Geometry: final body of the model. Coordinates: model frame, mm. A direction names the side the tool comes from. Give positions to 0.01 mm unless a question says otherwise; leave off trailing zeros. Write each loop counter-clockwise with the first axis right and the second up, starting at its lowest first coordinate (ties: lowest second). Pieces come first, ordered by that corner, then holes. Notation, with made-up numbers: M 15.5,80.5 L 65.5,80.5 A18 ccw 65.5,114.5 Z; hole C 26.25,48 d11. An arc over 180 degrees is marked long. Use one line per item in the form item = value. Start each with the question number.
Item 1: Contact query for flat-ended pins moving along their axis: P1, Ø1.5, axis at x = -25.5, y = -13.5, coming from the +Z side; P2, Ø8, axis at x = -6.5, y = -26.5, coming from the -Z side; P3, Ø3, axis at x = -5, y = -24, coming from the -Z side; P4, Ø1, axis at y = -25.5, z = -6.5, coming from the +X side. Output: stop coordinate, or through.
Item 2: Access query for faces 1 (the flat face through (-27, -12, 15)), 2 (the flat face through (-11, -20, -10)), 3 (the flat face through (-11, -20, -15)). Directions: +Z, -Z, +X, -X, +Y, -Y. A direction counts if a zero-diameter tool reaches every point of the face in a straight line with its end or side. Return the directions, or none.
Item 3: Section query D-D on y = -16. Return loops of the section in (x, z).
Item 4: Section query C-C on x = -25.5. Return loops of the section in (y, z).
Item 5: Section query A-A on y = -23. Return loops of the section in (x, z).
Item 6: Section query B-B on z = -12. Return loops of the section in (x, y).
Item 7: Material intervals for line 1 along Y through (x, z) = (16, 1); line 2 along X through (y, z) = (-17.5, -0.5); line 3 along Z through (x, y) = (-16.5, -13), sorted ascending. Write a range as from..to.
from build123d import *

# Parameters (mm, degrees)
F1_DEPTH = 10
F0_W     = 30
F0_H     = 5
F2_DEPTH = 35
F4_DEPTH = 10.001
F6_DEPTH = 10.001


with BuildPart() as f1:
    # F0 (on Front) → F1 (new body)
    with BuildSketch(Plane.XZ):
        Polygon((32.5, 0), (-7.5, 20), (-22.5, 20), (-32.5, 20), (-32.5, 15), (-22.5, 15), (-22.5, -10), (7.5, -10), (7.5, -15), (-22.5, -15), (-22.5, -20), (32.5, -20), align=None)
    extrude(amount=F1_DEPTH)

    # F0 (on Front) → F2 (join)
    with BuildSketch(Plane.XZ):
        Polygon((-22.5, 15), (-32.5, 15), (-32.5, 10), (-32.5, -20), (-22.5, -20), (-22.5, -15), (-22.5, -10), align=None)
        with Locations((-7.5, -12.5)):
            Rectangle(F0_W, F0_H)
    extrude(amount=F2_DEPTH)

    # F3 (on face) → F4 (cut, through all)
    with BuildSketch(Plane.XY.offset(-10)):
        Polygon((7.5, -10), (-22.5, -35), (7.5, -35), align=None)
    extrude(amount=-F4_DEPTH, mode=Mode.SUBTRACT)

    # F5 (on face) → F6 (cut, through all)
    with BuildSketch(Plane.YZ.offset(-22.5)):
        Polygon((-35, 15), (-35, 0), (-15, 15), align=None)
    extrude(amount=-F6_DEPTH, mode=Mode.SUBTRACT)


solid = f1.part
Answer sheet:
q1.P1 = 15
q1.P2 = -15
q1.P3 = through
q1.P4 = -22.5
q2.face_1 = +Z, +X, -X, -Y
q2.face_2 = +Z, +X, -Y
q2.face_3 = -Z, +X, -Y
q3.outline = M -32.5,-20 L -22.5,-20 L -22.5,-15 L 0.3,-15 L 0.3,-10 L -22.5,-10 L -22.5,14.25 L -32.5,14.25 Z
q4.outline = M -35,-20 L 0,-20 L 0,20 L -10,20 L -10,15 L -15,15 L -35,0 Z
q5.outline = M -32.5,-20 L -22.5,-20 L -22.5,-15 L -8.1,-15 L -8.1,-10 L -22.5,-10 L -22.5,9 L -32.5,9 Z
q6.outline = M -32.5,-35 L -22.5,-35 L 7.5,-10 L 32.5,-10 L 32.5,0 L -32.5,0 Z
q7.line_1 = -10..0
q7.line_2 = -32.5..-22.5
q7.line_3 = -15..-10
